Verification items for this drawing (mm, ordinates from the low corner). Coordinates: 2 decimals unless noted, no trailing zeros. Order: outer loops, then holes, each group sorted by start corner. A loop starts at its lowest first (then second) coordinate and runs counter-clockwise, first axis right, second up. Notation, with made-up numbers: (5.5, -35.75) -> (54.5, -35.75) arc R12 ccw to (54.5, -30.75) -> close; hole circle Ø8 at (7, -39). An arc over 180 degrees is marked (long way). Put each result on its own line as item: value. Start each with the question number.
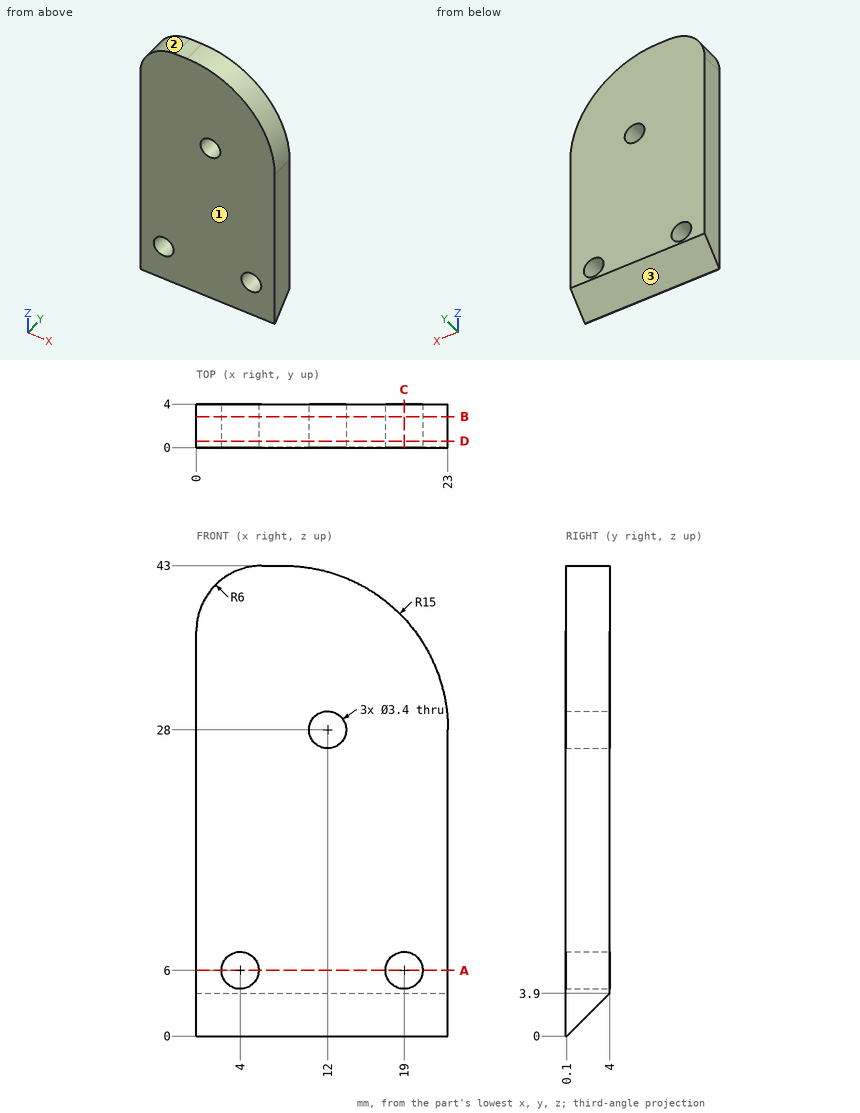
1) Mould release check, pull along Y, two halves, no side actions. Record for the marked faces 1, 2 and 3: +Y half, -Y half, draft (parallel to the pull), parting line (faces both ways), or undercut.
2) Sectioned sample at C-C (x = 19). Record the boundary of the cut face in (y, z).
3) Sectioned sample at A-A (z = 6). Record the boundary of the cut face in (x, y).
4) Gauge pin test, flat ends, axial feed: pin 1 (4.5 mm diameter, centred on x = 12, z = 28, fed in from +Y); pin 2 (1 mm diameter, centred on x = 8, y = 2, fed in from -Z). Record the tip position at first contact, or that the pin passes through.
5) Sectioned sample at B-B (y = 2.85). Record the boundary of the cut face in (x, z), plus the area to 4 significant figures.
6) Scan lines: line 1 along X through (y, z) = (2.9, 6); line 2 along Z through (x, y) = (19, 0.9); line 3 along Z through (x, y) = (12, 0.85). Record each from-to range of solid material in increasing order. Write a range as [from, to].
7) Sectioned sample at D-D (y = 0.6). Record the boundary of the cut face in (x, z), plus the area to 3 significant figures.
Entries:
1. face 1: -Y half
1. face 2: draft
1. face 3: +Y half
2. outline: (0, 0) -> (0.1, 0) -> (4, 3.9) -> (4, 4.3) -> (0, 4.3) -> close; (0, 7.7) -> (4, 7.7) -> (4, 38.2) -> (0, 38.2) -> close
3. outline: (0, 0) -> (2.3, 0) -> (2.3, 4) -> (0, 4) -> close; (5.7, 0) -> (17.3, 0) -> (17.3, 4) -> (5.7, 4) -> close; (20.7, 0) -> (23, 0) -> (23, 4) -> (20.7, 4) -> close
4. pin 1: stops at y = 4
4. pin 2: stops at z = 1.4
5. outline: (0, 2.75) -> (23, 2.75) -> (23, 28) arc R15 ccw to (8, 43) -> (6, 43) arc R6 ccw to (0, 37) -> close; hole circle Ø3.4 at (4, 6); hole circle Ø3.4 at (12, 28); hole circle Ø3.4 at (19, 6)
5. area: 842.5 mm2
6. line 1: x = [0, 2.3], [5.7, 17.3], [20.7, 23]
6. line 2: z = [0.8, 4.3], [7.7, 38.2]
6. line 3: z = [0.75, 26.3], [29.7, 42.46]
7. outline: (0, 0.5) -> (23, 0.5) -> (23, 28) arc R15 ccw to (8, 43) -> (6, 43) arc R6 ccw to (0, 37) -> close; hole circle Ø3.4 at (4, 6); hole circle Ø3.4 at (12, 28); hole circle Ø3.4 at (19, 6)
7. area: 894 mm2
